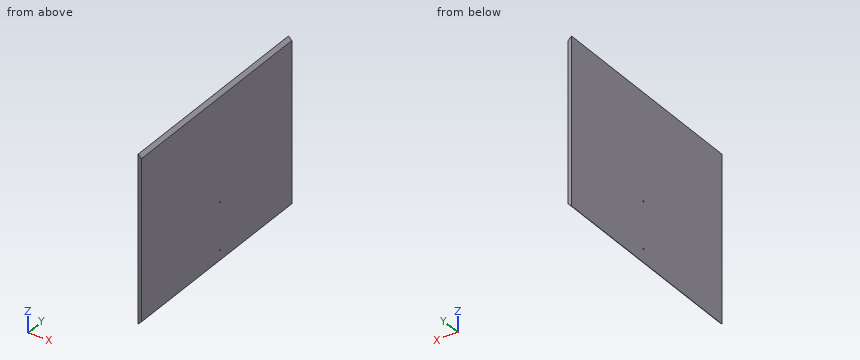
```python
from build123d import *

# Parameters (mm, degrees)
CROQUIS1_W              = 5
CROQUIS1_H              = 250
SALIENTE_EXTRUIR1_DEPTH = 330
CORTAR_EXTRUIR1_REACH   = 416.035
CORTAR_EXTRUIR2_REACH   = 416.035
CROQUIS6_R              = 1


with BuildPart() as part:
    # Croquis1 → Saliente-Extruir1 (new body)
    with BuildSketch(Plane(origin=(0, 0, 0), x_dir=(1, 0, 0), z_dir=(0, 1, 0))):
        with Locations((-2.5, 125)):
            Rectangle(CROQUIS1_W, CROQUIS1_H)
    extrude(amount=SALIENTE_EXTRUIR1_DEPTH)

    # Croquis2 → Cortar-Extruir1 (cut, up to next)
    with BuildSketch(Plane(origin=(0, 330, 0), x_dir=(1, 0, 0), z_dir=(0, 1, 0)), mode=Mode.PRIVATE) as cortar_extruir1_sk1:
        Polygon((0, 250), (0, 245), (-5, 250), align=None)
    cortar_extruir1_tool1 = extrude(cortar_extruir1_sk1.sketch, amount=-CORTAR_EXTRUIR1_REACH, mode=Mode.PRIVATE) & part.part
    # Croquis2 → Cortar-Extruir1 (cut, up to next)
    with BuildSketch(Plane(origin=(0, 330, 0), x_dir=(1, 0, 0), z_dir=(0, 1, 0)), mode=Mode.PRIVATE) as cortar_extruir1_sk2:
        Polygon((-5, 0), (0, 5), (0, 0), align=None)
    cortar_extruir1_tool2 = extrude(cortar_extruir1_sk2.sketch, amount=-CORTAR_EXTRUIR1_REACH, mode=Mode.PRIVATE) & part.part
    add(cortar_extruir1_tool1.solids().sort_by_distance((-1.666667, 330, -248.333333))[0], mode=Mode.SUBTRACT)
    add(cortar_extruir1_tool2.solids().sort_by_distance((-1.666667, 330, -1.666667))[0], mode=Mode.SUBTRACT)

    # Croquis6 → Cortar-Extruir2 (cut, up to next)
    with BuildSketch(Plane.ZY.offset(5), mode=Mode.PRIVATE) as cortar_extruir2_sk1:
        with Locations((-230, 172.2)):
            Circle(CROQUIS6_R)
    cortar_extruir2_tool1 = extrude(cortar_extruir2_sk1.sketch, amount=-CORTAR_EXTRUIR2_REACH, mode=Mode.PRIVATE) & part.part
    # Croquis6 → Cortar-Extruir2 (cut, up to next)
    with BuildSketch(Plane.ZY.offset(5), mode=Mode.PRIVATE) as cortar_extruir2_sk2:
        with Locations((-160, 172.2)):
            Circle(CROQUIS6_R)
    cortar_extruir2_tool2 = extrude(cortar_extruir2_sk2.sketch, amount=-CORTAR_EXTRUIR2_REACH, mode=Mode.PRIVATE) & part.part
    add(cortar_extruir2_tool1.solids().sort_by_distance((-5, 172.2, -230))[0], mode=Mode.SUBTRACT)
    add(cortar_extruir2_tool2.solids().sort_by_distance((-5, 172.2, -160))[0], mode=Mode.SUBTRACT)


solid = part.part
```
Verification items for the finished model (mm, model axes). Coordinates: 2 decimals unless noted, no trailing zeros. Write each loop counter-clockwise with the first axis right and the second up, starting at its lowest first coordinate (ties: lowest second). Pieces come first, ordered by that corner, then holes. Notation, with made-up numbers: (47.5, 21.5) - (89.5, 21.5) arc R30 cw to (89.5, 48.5) - close; hole circle Ø7 at (60, 0.5). An arc over 180 degrees is marked (long way). One line per question, with ' | ' between items. Start each with the question number.
1. Section check B-B (y = 194). Enter the section's corners in (x, z), plus the area to 4 significant figures.
2. Material ranges on line 1 along Y through (x, z) = (-2.7, -160); line 2 along Z through (x, y) = (-1.4, 172.2); line 3 along Z through (x, y) = (-2.65, 172.2), recorded low to high.
3. Gauge pin test, flat ends, axial feed: P1, Ø1, axis at x = -3.5, y = 277, coming from the +Z side; P2, Ø3, axis at x = -3, y = 46, coming from the +Z side; P3, Ø1.5, axis at x = -1.5, y = 142.5, coming from the +Z side. Record the tip position at first contact, or that the pin passes through.
4. Section check A-A (x = -1.85). Enter the section's corners in (y, z).
Computed values:
1) outline: (-5, -250) - (0, -245) - (0, -5) - (-5, 0) - close | area: 1,225 mm²
2) line 1: 0 to 171.2, 173.2 to 330 | line 2: -246.4 to -231, -229 to -161, -159 to -3.6 | line 3: -247.65 to -231, -229 to -161, -159 to -2.35
3) P1: z = -1 | P2: z = -0.5 | P3: z = -2.75
4) outline: (0, -246.85) - (330, -246.85) - (330, -3.15) - (0, -3.15) - close; hole circle Ø2 at (172.2, -230); hole circle Ø2 at (172.2, -160)
